from build123d import *

# Parameters (mm, degrees)
SKETCH1_W                = 40
SKETCH1_H                = 40
BOSS_EXTRUDE1_DEPTH      = 185
SKETCH2_R                = 7.5
BOSS_EXTRUDE2_DEPTH      = 20
BOSS_EXTRUDE2_DEPTH_BACK = 205


with BuildPart() as part:
    # Sketch1 → Boss-Extrude1 (new body)
    with BuildSketch(Plane(origin=(0, 0, 0), x_dir=(1, 0, 0), z_dir=(0, 1, 0))):
        Rectangle(SKETCH1_W, SKETCH1_H)
    extrude(amount=BOSS_EXTRUDE1_DEPTH)

    # Sketch2 → Boss-Extrude2 (add, two sides)
    with BuildSketch(Plane(origin=(0, 185, 0), x_dir=(1, 0, 0), z_dir=(0, 1, 0))) as boss_extrude2_sk:
        Circle(SKETCH2_R)
    extrude(amount=BOSS_EXTRUDE2_DEPTH)
    extrude(boss_extrude2_sk.sketch, amount=-BOSS_EXTRUDE2_DEPTH_BACK)


solid = part.part
Build history of the part. All positions in model axes, mm. A direction names the side the tool comes from. Round coordinates to 2 decimals unless told otherwise and drop trailing zeros. Write each loop counter-clockwise with the first axis right and the second up, starting at its lowest first coordinate (ties: lowest second). Pieces come first, ordered by that corner, then holes. Notation, with made-up numbers: M 22.25,80 L 63.25,80 A24 cw 63.25,95 Z; hole C 32,15.5 d7. An arc over 180 degrees is marked long. Use CSV: the item, a comma, the result in double quotes.
1. Tool access for faces 1 (the face through (-7.493, -9.86, -0.33)), 2 (the face through (-7.493, 194.86, -0.33)), 3 (the face through (0, 91, -20)): list every direction of +Z, -Z, +X, -X, +Y, -Y with a clear straight run to the whole face (end or side of a thin tool).
Reply:
face 1,"-Y"
face 2,"+Y"
face 3,"-Z, +X, -X, +Y, -Y"
2. Wall check: probe 1 along Y at (x, z) = (3, -16.5); probe 2 along X at (y, z) = (191.5, -2). Give the ranges that are in metal, low to high. Write a range as from..to.
Reply:
probe 1,"y = 0..185"
probe 2,"x = -7.23..7.23"
3. Saw through at C-C (z = 14). Give the cut face in (x, y).
Reply:
outline,"M -20,0 L 20,0 L 20,185 L -20,185 Z"
4. Saw through at A-A (x = 4.5). Give the cut face in (y, z).
Reply:
outline,"M -20,-6 L 0,-6 L 0,-20 L 185,-20 L 185,-6 L 205,-6 L 205,6 L 185,6 L 185,20 L 0,20 L 0,6 L -20,6 Z"
5. Saw through at B-B (z = 0). Give the cut face in (x, y).
Reply:
outline,"M -20,0 L -7.5,0 L -7.5,-20 L 7.5,-20 L 7.5,0 L 20,0 L 20,185 L 7.5,185 L 7.5,205 L -7.5,205 L -7.5,185 L -20,185 Z"
